```python
from build123d import *

# Parameters (mm, degrees)
SKETCH_1_R               = 12.5
EXTRUDE_1_DEPTH          = 2
SKETCH_2_R               = 1.65
CUT_EXTRUDE_1_DEPTH      = 18.790446875
PATTERN_CIRCULAR_1_COUNT = 6
SKETCH_6_R               = 7.5
CUT_EXTRUDE_3_DEPTH      = 18.790446875


with BuildPart() as part:
    # Эскиз1 → Бобышка-Вытянуть1 (new body)
    with BuildSketch(Plane(origin=(0, 0, 0), x_dir=(1, 0, 0), z_dir=(0, 1, 0))):
        with Locations(Location((0, 0, 0), (0, 0, 270))):
            Circle(SKETCH_1_R)
    extrude(amount=EXTRUDE_1_DEPTH)

    # Эскиз2 → Вырез-Вытянуть1 (cut, through all)
    with BuildSketch(Plane.XZ):
        with Locations(Location((0, -10.176132167, 0), (0, 0, 270))):
            Circle(SKETCH_2_R)
    cut_extrude_1 = extrude(amount=-CUT_EXTRUDE_1_DEPTH, mode=Mode.SUBTRACT)

    # Круговой массив1: Вырез-Вытянуть1 ×6 about axis
    pattern_circular_1_axis = Axis((0, 0, 0), (0, 1, 0))
    for i in range(1, PATTERN_CIRCULAR_1_COUNT):
        add(cut_extrude_1.rotate(pattern_circular_1_axis, i * 360 / PATTERN_CIRCULAR_1_COUNT), mode=Mode.SUBTRACT)

    # Эскиз6 → Вырез-Вытянуть3 (cut, through all)
    with BuildSketch(Plane(origin=(0, 2, 0), x_dir=(1, 0, 0), z_dir=(0, 1, 0))):
        with Locations(Location((0, 0, 0), (0, 0, 270))):
            Circle(SKETCH_6_R)
    extrude(amount=-CUT_EXTRUDE_3_DEPTH, mode=Mode.SUBTRACT)


solid = part.part
```
For this review, take the finished solid that the model builds, in its own axes (mm). Round coordinates to 2 decimals unless told otherwise and drop trailing zeros. Write each loop counter-clockwise with the first axis right and the second up, starting at its lowest first coordinate (ties: lowest second). Pieces come first, ordered by that corner, then holes.
1) Take a section at A-A on z = 0. Give the boundary of the cut face in (x, y).
Answer below:
outline: (-12.5, 0) - (-7.5, 0) - (-7.5, 2) - (-12.5, 2) - close; (7.5, 0) - (12.5, 0) - (12.5, 2) - (7.5, 2) - close
2) Take a section at B-B on x = 0. Give the boundary of the cut face in (y, z), then the cut area to 3 significant figures.
Answer below:
outline: (0, -12.5) - (2, -12.5) - (2, -11.83) - (0, -11.83) - close; (0, -8.53) - (2, -8.53) - (2, -7.5) - (0, -7.5) - close; (0, 7.5) - (2, 7.5) - (2, 8.53) - (0, 8.53) - close; (0, 11.83) - (2, 11.83) - (2, 12.5) - (0, 12.5) - close
area: 6.80 mm2
3) For line 1 along X through (y, z) = (0.8, -5.5); line 2 along Z through (x, y) = (1, 1.65); line 3 along Z through (x, y) = (5.25, 1.9), list the stretches that pass through material, from the lowest coordinate up.
Answer below:
line 1: x = -11.22 to -10.41, -7.22 to -5.1, 5.1 to 7.22, 10.41 to 11.22
line 2: z = -12.46 to -11.49, -8.86 to -7.43, 7.43 to 8.86, 11.49 to 12.46
line 3: z = -11.34 to -5.36, 5.36 to 11.34
4) Take a section at C-C on y = 1. Give the boundary of the cut face in (x, z), then the cut area to 3 significant figures.
Answer below:
outline: circle Ø25 at (0, 0); hole circle Ø3.3 at (-8.81, -5.09); hole circle Ø3.3 at (-8.81, 5.09); hole circle Ø15 at (0, 0); hole circle Ø3.3 at (0, -10.18); hole circle Ø3.3 at (0, 10.18); hole circle Ø3.3 at (8.81, -5.09); hole circle Ø3.3 at (8.81, 5.09)
area: 263 mm2
5) Mouldability with a two-part tool opening along X and no side actions: class faces 1 (the face through (-8, 0, 0)), 2 (the face through (-7.42, 0.99, 4.2)), 3 (the face through (3.755, 0.986, 11.923)) as +X half, -X half, draft (parallel to the pull), parting line (faces both ways), or undercut.
Answer below:
face 1: draft
face 2: undercut
face 3: parting line
6) Take a section at D-D on z = 4. Give the boundary of the cut face in (x, y), then the cut area to 3 significant figures.
Answer below:
outline: (-11.84, 0) - (-10.05, 0) - (-10.05, 2) - (-11.84, 2) - close; (-7.57, 0) - (-6.34, 0) - (-6.34, 2) - (-7.57, 2) - close; (6.34, 0) - (7.57, 0) - (7.57, 2) - (6.34, 2) - close; (10.05, 0) - (11.84, 0) - (11.84, 2) - (10.05, 2) - close
area: 12.1 mm2
